CAD build for the part. Positions are in the model's coordinates, mm. A direction names the side the tool comes from. Coordinates: 2 decimals unless noted, no trailing zeros. Loops run counter-clockwise (first coordinate to the right, second up) from the corner with the lowest first, then second, coordinate; pieces in that order, holes last. Notation, with made-up numbers: (74.5, 52.5) -> (94.5, 52.5) arc R11 ccw to (94.5, 63.5) -> close; hole circle Ø3 at (73.5, 42). An arc over 180 degrees is marked (long way). Write each question's results on one line, items separated by ' | '.
from build123d import *

# Parameters (mm, degrees)
SKETCH1_W           = 39.6
SKETCH1_H           = 39.6
BOSS_EXTRUDE1_DEPTH = 7
SHELL2_T            = -0.2
CUT_EXTRUDE1_DEPTH  = 8


with BuildPart() as part:
    # Sketch1 → Boss-Extrude1 (new body)
    with BuildSketch(Plane(origin=(0, 0, 0), x_dir=(1, 0, 0), z_dir=(0, 1, 0))):
        Rectangle(SKETCH1_W, SKETCH1_H)
    extrude(amount=BOSS_EXTRUDE1_DEPTH)

    # Shell2
    shell2_openings = [part.faces().sort_by_distance(p)[0] for p in [
        (0, 0, 0),
    ]]
    offset(amount=SHELL2_T, openings=shell2_openings, kind=Kind.INTERSECTION)

    # Sketch2 → Cut-Extrude1 (cut, through all)
    with BuildSketch(Plane(origin=(0, 0, 0), x_dir=(1, 0, 0), z_dir=(0, 1, 0))):
        with BuildLine():
            Line((17.55, -18.3), (0.75, -18.3))
            Line((0.75, -18.3), (0.75, -2.90473751))
            ThreePointArc((0.75, -2.90473751), (2.121320344, -2.121320344), (2.90473751, -0.75))
            Line((2.90473751, -0.75), (18.3, -0.75))
            Line((18.3, -0.75), (18.3, -17.55))
            Line((18.3, -17.55), (17.55, -18.3))
        make_face()
        with BuildLine():
            Line((17.55, 18.3), (0.75, 18.3))
            Line((0.75, 18.3), (0.75, 2.90473751))
            ThreePointArc((0.75, 2.90473751), (2.121320344, 2.121320344), (2.90473751, 0.75))
            Line((2.90473751, 0.75), (18.3, 0.75))
            Line((18.3, 0.75), (18.3, 17.55))
            Line((18.3, 17.55), (17.55, 18.3))
        make_face()
        with BuildLine():
            Line((-18.3, -17.55), (-18.3, -0.75))
            Line((-18.3, -0.75), (-2.90473751, -0.75))
            ThreePointArc((-2.90473751, -0.75), (-2.121320344, -2.121320344), (-0.75, -2.90473751))
            Line((-0.75, -2.90473751), (-0.75, -18.3))
            Line((-0.75, -18.3), (-17.55, -18.3))
            Line((-17.55, -18.3), (-18.3, -17.55))
        make_face()
        with BuildLine():
            Line((-0.75, 18.3), (-0.75, 2.90473751))
            ThreePointArc((-0.75, 2.90473751), (-2.121320344, 2.121320344), (-2.90473751, 0.75))
            Line((-2.90473751, 0.75), (-18.3, 0.75))
            Line((-18.3, 0.75), (-18.3, 17.55))
            Line((-18.3, 17.55), (-17.55, 18.3))
            Line((-17.55, 18.3), (-0.75, 18.3))
        make_face()
    extrude(amount=CUT_EXTRUDE1_DEPTH, mode=Mode.SUBTRACT)


solid = part.part
1) Slice it at B-B (y = 4.75). Write the cut outline in (x, z).
Outcome:
outline: (-19.8, -19.8) -> (19.8, -19.8) -> (19.8, 19.8) -> (-19.8, 19.8) -> close; hole (-19.6, -19.6) -> (19.6, -19.6) -> (19.6, 19.6) -> (-19.6, 19.6) -> close
2) Drill centre lines: L1, parallel to X at y = 3.75, z = 3; L2, parallel to Y at x = -10, z = 0. Where is each one in solid material? Low to high. Write a range as from..to.
Outcome:
L1: x = -19.8..-19.6, 19.6..19.8 | L2: y = 6.8..7
3) Slice it at C-C (z = 12). Write the cut outline in (x, y).
Outcome:
outline: (-19.8, 0) -> (-19.6, 0) -> (-19.6, 6.8) -> (-18.3, 6.8) -> (-18.3, 7) -> (-19.8, 7) -> close; (-0.75, 6.8) -> (0.75, 6.8) -> (0.75, 7) -> (-0.75, 7) -> close; (18.3, 6.8) -> (19.6, 6.8) -> (19.6, 0) -> (19.8, 0) -> (19.8, 7) -> (18.3, 7) -> close
4) Pin check, flat tips, straight feed: pin 1 (12 mm diameter, centred on x = -8, z = -4, fed in from -Y); pin 2 (1 mm diameter, centred on x = -10, z = 2.5, fed in from +Y). Stop position of each tip, or through.
Outcome:
pin 1: stops at y = 6.8 | pin 2: passes through
5) Slice it at A-A (x = -11.5). Write the cut outline in (y, z).
Outcome:
outline: (0, -19.8) -> (7, -19.8) -> (7, -18.3) -> (6.8, -18.3) -> (6.8, -19.6) -> (0, -19.6) -> close; (0, 19.6) -> (6.8, 19.6) -> (6.8, 18.3) -> (7, 18.3) -> (7, 19.8) -> (0, 19.8) -> close; (6.8, -0.75) -> (7, -0.75) -> (7, 0.75) -> (6.8, 0.75) -> close
6) Which spindle directions (+Z, -Z, +X, -X, +Y, -Y) get a long thin tool onto all of the face, cutting with end or side? Do faces 1 (the flat face through (-19.6, 3, 0)), 2 (the flat face through (0, 3, -19.8)). Say none if no direction does.
Outcome:
face 1: -Y | face 2: -Z, +X, -X, +Y, -Y
7) Two-plate mould, pull along X, no slides. Class faces 3 (the flat face through (0, 3, 19.8)), 4 (the flat face through (0, 3, 19.6)), 5 (the flat face through (-19.8, 3, 0)), 6 (the flat face through (19.6, 3, 0)): pulls with the +X half, pulls with the -X half, needs draft (parallel to the pull), parting line crosses it, or undercut.
Outcome:
face 3: needs draft | face 4: undercut | face 5: pulls with the -X half | face 6: undercut
